Could you check a few things on this model? Use its own coordinates, in mm. A direction names the side the tool comes from. Coordinates: 2 decimals unless noted, no trailing zeros. Write each loop counter-clockwise with the first axis right and the second up, starting at its lowest first coordinate (ties: lowest second). Pieces come first, ordered by that corner, then holes. Notation, with made-up numbers: M 80.5,-29.5 L 115.5,-29.5 A31 cw 115.5,8.5 Z; hole C -30,-6 d8. An arc over 180 degrees is marked long. Answer as CSV lines item,"result". Start each with the question number.
Item 1: We'd pull the mould along X, two halves only. Please class faces 1 (the cylindrical face through (28, -4, -45)), 2 (the cylindrical face through (-4.868, -4.056, 87.349)), 3 (the cylindrical face through (-289.319, 96.056, 168.876)), 4 (the cylindrical face through (279.487, 95.944, 0.565)): +X half, -X half, draft (parallel to the pull), parting line (faces both ways), or undercut.
Item 2: On a 3-axis mill with a long thin cutter (end or side, diameter ignored), from which of +Z, -Z, +X, -X, +Y, -Y can I reach the whole of each face in a straight line? I mean faces 5 (the flat face through (-50, 0, 24)), 6 (the cylindrical face through (-279.487, 95.944, -0.565)), 7 (the flat face through (-262, 92, -147)), 8 (the flat face through (255, 92, -150)), 9 (the flat face through (1, -8, 177)). Say none if no direction works.
Item 3: If I drill on line 1 along X through (y, z) = (-2, -81); line 2 along X through (y, z) = (-2.5, -40.5); line 3 along X through (y, z) = (-3, 0), over which ranges is the centre line in solid material (lowest first)? Write a range as [from, to].
Item 4: Suppose I cut it at A-A, the plane y = 47.5. Write out the boundary of the cut face in (x, z).
Item 5: I'm going to push flat-ended pins straight in: P1, Ø5, axis at y = -15.5, z = 0.5, coming from the +X side; P2, Ø5, axis at x = -62, y = 32.5, coming from the -Z side; P3, Ø1.5, axis at y = -3, z = 3.5, coming from the +X side. Where does each tip first touch, or does it pass through?
```python
from build123d import *

# Parameters (mm, degrees)
THICKEN1_T1        = 8
CUT_EXTRUDE1_DEPTH = 10
CIRPATTERN1_COUNT  = 6
SKETCH3_R          = 8
CUT_EXTRUDE2_DEPTH = 10
CIRPATTERN2_COUNT  = 6


with BuildPart() as body_1:
    # Surface-Revolve1: a surface, the sketch's curves turned about an axis
    with BuildLine(Plane.XY, mode=Mode.PRIVATE) as surface_revolve1_1_path:
        Line((53, 0), (116, 0))
        ThreePointArc((116, 0), (143.354158733, -20.5), (170.708317466, 0))
        Line((170.708317466, 0), (200.708317466, 0))
        ThreePointArc((200.708317466, 0), (221.905088036, 6.078076154), (236.660079318, 22.465154128))
        Line((236.660079318, 22.465154128), (274.476350399, 100))
        Line((274.476350399, 100), (335, 100))
    surface_revolve1_1 = Shell.revolve(surface_revolve1_1_path.wire(), 360, Axis((0, 0, 0), (0, 1, 0)))
    add(Solid.thicken(surface_revolve1_1, THICKEN1_T1))

    # Sketch2 → Cut-Extrude1 (cut)
    with BuildSketch(Plane.XZ.offset(-92)):
        with BuildLine():
            ThreePointArc((-278.640810912, 185.968541679), (-138.384551206, 242.808900604), (-18, 334.516068373))
            ThreePointArc((-18, 334.516068373), (-165.878071475, 291.048905519), (-278.640810912, 185.968541679))
        make_face()
        with BuildLine():
            ThreePointArc((0, 325), (-10, 315), (0, 305))
            Line((0, 305), (0, 325))
        make_face()
        with BuildLine():
            Line((0, 325), (0, 305))
            ThreePointArc((0, 305), (7.071067812, 307.928932188), (10, 315))
            ThreePointArc((10, 315), (7.071067812, 322.071067812), (0, 325))
        make_face()
    cut_extrude1 = extrude(amount=-CUT_EXTRUDE1_DEPTH, mode=Mode.SUBTRACT)

    # CirPattern1: Cut-Extrude1 ×6 about axis
    cirpattern1_axis = Axis((0, 0, 0), (0, 1, 0))
    for i in range(1, CIRPATTERN1_COUNT):
        add(cut_extrude1.rotate(cirpattern1_axis, i * 360 / CIRPATTERN1_COUNT), mode=Mode.SUBTRACT)

    # Sketch3 → Cut-Extrude2 (cut)
    with BuildSketch(Plane.XZ.offset(8)):
        with Locations(Location((0, 81, 0), (0, 0, 270))):
            Circle(SKETCH3_R)
    cut_extrude2 = extrude(amount=-CUT_EXTRUDE2_DEPTH, mode=Mode.SUBTRACT)

    # CirPattern2: Cut-Extrude2 ×6 about axis
    cirpattern2_axis = Axis((0, 0, 0), (0, 1, 0))
    for i in range(1, CIRPATTERN2_COUNT):
        add(cut_extrude2.rotate(cirpattern2_axis, i * 360 / CIRPATTERN2_COUNT), mode=Mode.SUBTRACT)


solid = body_1.part
```
Ans:
1,face 1,"undercut"
1,face 2,"undercut"
1,face 3,"-X half"
1,face 4,"+X half"
2,face 5,"+Y"
2,face 6,"-X, +Y, -Y"
2,face 7,"-Z, -X, -Y"
2,face 8,"-Z, +X, -Y"
2,face 9,"-Y"
3,line 1,"x = [-208.78, -149.51], [-83.96, -8], [8, 83.96], [149.51, 208.78]"
3,line 2,"x = [-219.31, -164.95], [-109.62, -78.15], [-62.15, -34.19], [34.19, 62.15], [78.15, 109.62], [164.95, 219.31]"
3,line 3,"x = [-222.04, -169.65], [-117.06, -53], [53, 117.06], [169.65, 222.04]"
4,outline,"C 0,0 d515.54; hole C 0,0 d497.74"
5,P1,"stops at x = 173.21"
5,P2,"stops at z = -244.07"
5,P3,"stops at x = 223.46"
